Read the model definition and answer for the solid it produces. Units are mm, in the model's axes. Face numbers are marked on the shaded views. A direction names the side the tool comes from. Coordinates: 2 decimals unless noted, no trailing zeros. Write each loop counter-clockwise with the first axis right and the second up, starting at its lowest first coordinate (ties: lowest second). Pieces come first, ordered by that corner, then holes. Notation, with made-up numbers: (88, -34) -> (129, -34) arc R5 cw to (129, -30) -> close; hole circle Ø5 at (9.25, 88). An arc over 180 degrees is marked (long way). Return JSON: item names as keys, results as strings.
from build123d import *

# Parameters (mm, degrees)
ESQUISSE1_R             = 6.75
ESQUISSE1_R_2           = 3
EXTRUSION1_DEPTH        = 4.5
CHANFREIN1_SIZE         = 2
CHANFREIN1_SIZE2        = 1.154700538
ENL_V_START             = -4.500004
ENL_V_MAT_EXTRU_1_DEPTH = 4.500004
CHANFREIN3_SIZE         = 0.5
ESQUISSE7_W             = 0.625
ESQUISSE7_H             = 6.25
ENL_V_MAT_EXTRU_3_REACH = 8.25
ESQUISSE8_R             = 1.75
ESQUISSE9_R             = 1.75
ESQUISSE9_R_2           = 0.75
EXTRUSION2_DEPTH        = 2
CHANFREIN4_SIZE         = 1
ESQUISSE10_R            = 3
ENL_V_MAT_EXTRU_4_DEPTH = 5.5000001


with BuildPart() as part:
    # Esquisse1 → Extrusion1 (new body)
    with BuildSketch(Plane.XY):
        Circle(ESQUISSE1_R)
        Circle(ESQUISSE1_R_2, mode=Mode.SUBTRACT)
    extrude(amount=EXTRUSION1_DEPTH)

    # Chanfrein1
    chanfrein1_edges = [part.edges().sort_by_distance(p)[0] for p in [
        (-6.75, 0, 0),
    ]]
    chanfrein1_side = [part.faces().sort_by_distance(p)[0] for p in [
        (-6.559081169, 0, 0),
    ]]
    chamfer(chanfrein1_edges, length=CHANFREIN1_SIZE, length2=CHANFREIN1_SIZE2, reference=chanfrein1_side[0])

    # Esquisse3 → Enlèv. mat.-Extru.1 (cut)
    with BuildSketch(Plane.XY.offset(4.5).offset(ENL_V_START)):
        with BuildLine():
            Line((-0.5, 6.731456009), (-0.5, -5))
            Line((-0.5, -5), (0.5, -5))
            Line((0.5, -5), (0.5, 6.731456009))
            ThreePointArc((0.5, 6.731456009), (0, 6.75), (-0.5, 6.731456009))
        make_face()
    extrude(amount=ENL_V_MAT_EXTRU_1_DEPTH, mode=Mode.SUBTRACT)

    # Chanfrein3
    chanfrein3_edges = [part.edges().sort_by_distance(p)[0] for p in [
        (-4.592793268, -4.946589734, 4.5),
    ]]
    chamfer(chanfrein3_edges, length=CHANFREIN3_SIZE)

    # Esquisse7 → Trou taraudé M1.61 (revolve, cut)
    with BuildSketch(Plane(origin=(-0.5, 4.481456009, 2.25), x_dir=(0, 0, -1), z_dir=(0, 1, 0))):
        with Locations((0.3125, 3.125)):
            Rectangle(ESQUISSE7_W, ESQUISSE7_H)
    revolve(axis=Axis((5.85, 4.481456009, 2.25), (-1, 0, 0)), mode=Mode.SUBTRACT)

    # Esquisse8 → Enlèv. mat.-Extru.3 (cut, up to next)
    with BuildSketch(Plane.ZY.offset(-0.5), mode=Mode.PRIVATE) as enl_v_mat_extru_3_sk1:
        with Locations((2.25, 4.481456009)):
            Circle(ESQUISSE8_R)
    enl_v_mat_extru_3_tool1 = extrude(enl_v_mat_extru_3_sk1.sketch, amount=-ENL_V_MAT_EXTRU_3_REACH, mode=Mode.PRIVATE) & part.part
    add(enl_v_mat_extru_3_tool1.solids().sort_by_distance((0.5, 4.481456, 2.25))[0], mode=Mode.SUBTRACT)

    # Esquisse9 → Extrusion2 (add)
    with BuildSketch(Plane.ZY.offset(-0.5)):
        with Locations((2.25, 4.481456009)):
            Circle(ESQUISSE9_R)
        with Locations((2.25, 4.481456009)):
            Circle(ESQUISSE9_R_2, mode=Mode.SUBTRACT)
    extrude(amount=-EXTRUSION2_DEPTH)

    # Chanfrein4
    chanfrein4_edges = [part.edges().sort_by_distance(p)[0] for p in [
        (-3, 0, 4.5),
        (3, 0, 4.5),
    ]]
    chamfer(chanfrein4_edges, length=CHANFREIN4_SIZE)

    # Esquisse10 → Enlèv. mat.-Extru.4 (cut, through all)
    with BuildSketch(Plane.XY.offset(4.5)):
        Circle(ESQUISSE10_R)
    extrude(amount=-ENL_V_MAT_EXTRU_4_DEPTH, mode=Mode.SUBTRACT)


solid = part.part
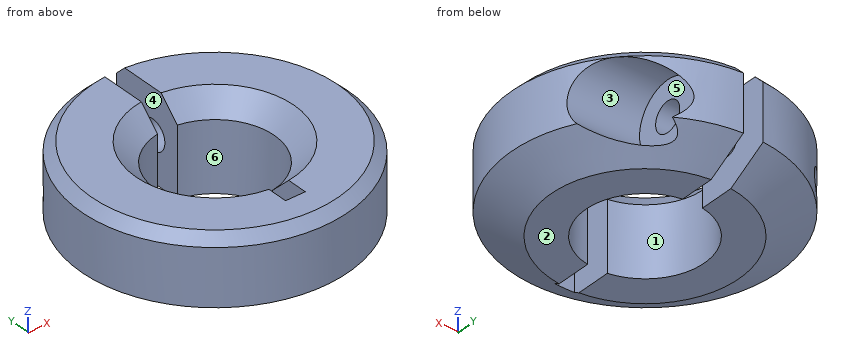
1. The part is cut by section D-D (x = 1.75). Count the separate pieces of the cut face and the enclosed holes in it, then the cut area to 3 significant figures.
Taken from the geometry:
{"separate pieces": "2", "enclosed holes": "1", "area": "31.1 mm2"}
2. The part is cut by section A-A (y = 0). Determine the outline of the cut face in (x, z), then the cut area to 3 significant figures.
Taken from the geometry:
{"outline": "(-6.75, 1.15) -> (-4.75, 0) -> (-3, 0) -> (-3, 3.5) -> (-4, 4.5) -> (-6.25, 4.5) -> (-6.75, 4) -> close; (3, 0) -> (4.75, 0) -> (6.75, 1.15) -> (6.75, 4) -> (6.25, 4.5) -> (4, 4.5) -> (3, 3.5) -> close", "area": "30.2 mm2"}
3. A tool of negligible diameter and unlimited length cuts with its end or side. For the marked faces 4, 5 and 6, from which of +Z, -Z, +X, -X, +Y, -Y can it reach the whole face along a straight path? Write none if from no direction.
Taken from the geometry:
{"face 4": "+Z, -Z, +Y", "face 5": "+X", "face 6": "+Z, -Z"}
4. The part is cut by section C-C (x = 0). Determine the outline of the cut face in (y, z), then the cut area to 3 significant figures.
Taken from the geometry:
{"outline": "(-6.75, 1.15) -> (-5, 0.14) -> (-5, 4.5) -> (-6.25, 4.5) -> (-6.75, 4) -> close", "area": "6.61 mm2"}
5. Consider L1, parallel to Y at x = 1.65, z = 2.25; L2, parallel to Y at x = 1.6, z = 2.25; L3, parallel to X at y = 4.5, z = 1.2. Determine where each line is inside the solid, lowest interval first.
Taken from the geometry:
{"L1": "y = -6.55 to -2.51, 2.51 to 3.73, 5.23 to 6.55", "L2": "y = -6.56 to -2.54, 2.54 to 3.73, 5.23 to 6.56", "L3": "x = -5.03 to -0.5, 0.5 to 2.5"}
6. The part is cut by section B-B (z = 2.25). Determine the outline of the cut face in (x, y), then the cut area to 3 significant figures.
Taken from the geometry:
{"outline": "(-5.54, 3.86) arc R6.75 ccw (long way) to (6.17, 2.73) -> (2.5, 2.73) -> (2.5, 3.73) -> (0.5, 3.73) -> (0.5, 2.96) arc R3 cw to (0.5, -2.96) -> (0.5, -5) -> (-0.5, -5) -> (-0.5, -2.96) arc R3 cw to (-0.5, 2.96) -> (-0.5, 3.86) -> close; (-4.41, 5.11) -> (-0.5, 5.11) -> (-0.5, 6.73) arc R6.75 ccw to start; (0.5, 5.23) -> (2.5, 5.23) -> (2.5, 6.23) -> (2.59, 6.23) arc R6.75 ccw to (0.5, 6.73) -> close", "area": "92.2 mm2"}
7. Flat-ended cylindrical pins translate along their axes: pin 1 Ø8 at (x, y) = (-1, -2) entering from -Z; pin 2 Ø0.8 at (y, z) = (4.48, 2.25) entering from +X; pin 3 Ø2 at (y, z) = (-4.5, 2.5) entering from -X; pin 4 Ø2 at (y, z) = (-3.5, 2) entering from +X. Find the tip coordinate at first contact, or state that the pin passes through.
Taken from the geometry:
{"pin 1": "stops at z = 0", "pin 2": "passes through", "pin 3": "stops at x = -5.77", "pin 4": "stops at x = 6.27"}
8. For a pull along Z with two mould halves and no side action, classify the marked faces 1, 2 and 3 as +Z half, -Z half, draft (parallel to the pull), parting line (faces both ways), or undercut.
Taken from the geometry:
{"face 1": "draft", "face 2": "-Z half", "face 3": "undercut"}
